Build history of the part. All positions in model axes, mm. A direction names the side the tool comes from. Coordinates: 2 decimals unless noted, no trailing zeros. Loops run counter-clockwise (first coordinate to the right, second up) from the corner with the lowest first, then second, coordinate; pieces in that order, holes last.
Item 1: Cut at D-D (x = 8). List the corners of the cut face in (y, z).
Item 2: Flat gauge pins, fed straight in: pin 1 (1.8 mm diameter, centred on x = 5, z = 10.5, fed in from -Y); pin 2 (5 mm diameter, centred on x = -10.5, y = -11.5, fed in from +Z); pin 3 (8 mm diameter, centred on y = -18.5, z = 16.5, fed in from +X); pin 4 (5.5 mm diameter, centred on x = -4, z = 17, fed in from -Y). Where does each tip first touch, or does it go through?
Item 3: Mould opens along Z. For faces 1 (the face through (-21.53, -2.22, 21.5)), 2 (the face through (-22.5, -10, 14)), 3 (the face through (-4.8, -11.3, 12)), 4 (the face through (-9, -3, 17)) say: released by +Z, released by -Z, zero draft, split by the parting line, or undercut.
Item 4: Drill centre lines: line 1 along Z through (x, y) = (-11, -12); line 2 along Z through (x, y) = (13.5, -1.5); line 3 along Z through (x, y) = (-18.5, -3.25). Where is each one in solid material? Low to high.
Item 5: 3-axis set-ups, long thin cutter, end or side, ignore diameter. For faces 5 (the face through (-14.04, -2.26, 19.67)), 6 (the face through (-12, -3, 24.164)), 7 (the face through (4.31, -14.62, 9.55)), 8 (the face through (-14, -11, 15.164)), 9 (the face through (0, -3, 19)): which of +Z, -Z, +X, -X, +Y, -Y reach the whole face in a straight line?
Item 6: Cut at C-C (z = 16.75). List the corners of the cut face in (x, y), and give its area (3 significant figures).
Item 7: Cut at B-B (y = -14.5). List the corners of the cut face in (x, z).
Item 8: Cut at A-A (x = -16). List the corners of the cut face in (y, z), and give its area (3 significant figures).
from build123d import *

# Parameters (mm, degrees)
F1_DEPTH  = 6
F2_DEPTH  = 23
F3_DEPTH  = 6
F4_R      = 5
F5_W      = 0.81186831
F5_H      = 2
F6_REACH  = 31.1431356237
F8_DEPTH  = 2
F10_DEPTH = 2
F11_R     = 5


with BuildPart() as f1:
    # F0 (on Front) → F1 (new body)
    with BuildSketch(Plane.XZ):
        with BuildLine():
            ThreePointArc((0, 22.7640915698), (-0.4760169509, 23.6848881741), (-1.3951592846, 24.1640915698))
            Line((-1.3951592846, 24.1640915698), (-22.5, 24.1640915698))
            ThreePointArc((-22.5, 24.1640915698), (-21.5061278282, 21.4707603394), (-18.9498743711, 20.1640915698))
            Line((-18.9498743711, 20.1640915698), (-9, 19.1640915698))
            Line((-9, 19.1640915698), (-9, 15.1640915698))
            Line((-9, 15.1640915698), (-6.2313233502, 15.1640915698))
            ThreePointArc((-6.2313233502, 15.1640915698), (-1.9506759829, 13.9418160027), (1.7829414728, 11.5173572715))
            ThreePointArc((1.7829414728, 11.5173572715), (0.6303147693, 13.2130414674), (0, 15.1640915698))
            Line((0, 15.1640915698), (0, 22.7640915698))
        make_face()
    extrude(amount=F1_DEPTH)

    # F0 (on Front) → F2 (join)
    with BuildSketch(Plane.XZ):
        with BuildLine():
            ThreePointArc((2.5376606134, 10.8007404291), (2.1473911285, 11.1454525194), (1.7829414728, 11.5173572715))
            ThreePointArc((1.7829414728, 11.5173572715), (-1.9506759829, 13.9418160027), (-6.2313233502, 15.1640915698))
            Line((-6.2313233502, 15.1640915698), (-9, 15.1640915698))
            Line((-9, 15.1640915698), (-22.5, 15.1640915698))
            Line((-22.5, 15.1640915698), (-22.5, 13.1640915698))
            Line((-22.5, 13.1640915698), (-11, 13.1640915698))
            ThreePointArc((-11, 13.1640915698), (-3.8410894684, 11.591731055), (2, 7.1640915698))
            Line((2, 7.1640915698), (20.2497988939, 7.1640915698))
            Line((20.2497988939, 7.1640915698), (20.2497988939, 9.1640915698))
            Line((20.2497988939, 9.1640915698), (7.4160159886, 9.1640915698))
            ThreePointArc((7.4160159886, 9.1640915698), (7.1261843392, 9.1582804924), (6.8363526899, 9.1640915698))
            Line((6.8363526899, 9.1640915698), (3.930054605, 9.1640915698))
            ThreePointArc((3.930054605, 9.1640915698), (3.2631933631, 10.0073736605), (2.5376606134, 10.8007404291))
        make_face()
    extrude(amount=F2_DEPTH)

    # F0 (on Front) → F3 (join)
    with BuildSketch(Plane.XZ):
        with BuildLine():
            ThreePointArc((6.8363526899, 9.1640915698), (4.5533954509, 9.6314834175), (2.5376606134, 10.8007404291))
            ThreePointArc((2.5376606134, 10.8007404291), (3.2631933631, 10.0073736605), (3.930054605, 9.1640915698))
            Line((3.930054605, 9.1640915698), (6.8363526899, 9.1640915698))
        make_face()
    extrude(amount=F3_DEPTH)

    # F4
    f4_edges = [f1.edges().sort_by_distance(p)[0] for p in [
        (3.930055, -14.5, 9.164092),
    ]]
    fillet(f4_edges, radius=F4_R)

    f6_end = Plane(origin=(-13.9749371855, -3, 19.6640915698), x_dir=(-0.9949874371, 0, 0.1), z_dir=(-0.1, 0, -0.9949874371))
    # F5 (on face) → F6 (cut, up to a plane its end follows)
    with BuildSketch(Plane.XY.offset(24.1640915698)):
        Polygon((-8.5, -6), (-22.5, -4), (-22.5, -6), align=None)
        with Locations((-22.905934155, -5)):
            Rectangle(F5_W, F5_H)
    f6_long = extrude(amount=-F6_REACH, mode=Mode.PRIVATE)
    add(split(f6_long, bisect_by=f6_end, keep=Keep.BOTTOM, mode=Mode.PRIVATE), mode=Mode.SUBTRACT)

    # F7 (on face) → F8 (cut, through all)
    with BuildSketch(Plane.XY.offset(15.1640915698)):
        with BuildLine():
            ThreePointArc((-19.6606274694, -23), (-21.6815784663, -21.9369160005), (-22.5, -19.8051147163))
            Line((-22.5, -19.8051147163), (-22.5, -23))
            Line((-22.5, -23), (-19.6606274694, -23))
        make_face()
    extrude(amount=-F8_DEPTH, mode=Mode.SUBTRACT)

    # F9 (on face) → F10 (cut, through all)
    with BuildSketch(Plane.XY.offset(9.1640915698)):
        with BuildLine():
            ThreePointArc((20.2497988939, -21.1107209325), (19.5387380379, -22.4279634054), (18.1554414653, -23))
            Line((18.1554414653, -23), (20.2497988939, -23))
            Line((20.2497988939, -23), (20.2497988939, -21.1107209325))
        make_face()
    extrude(amount=-F10_DEPTH, mode=Mode.SUBTRACT)

    # F11
    f11_edges = [f1.edges().sort_by_distance(p)[0] for p in [
        (2, -11.5, 7.164092),
    ]]
    fillet(f11_edges, radius=F11_R)


solid = f1.part
Filled sheet:
1. outline: (-23, 7.16) - (0, 7.16) - (0, 9.16) - (-23, 9.16) - close
2. pin 1: passes through
2. pin 2: stops at z = 15.16
2. pin 3: stops at x = 0.55
2. pin 4: stops at y = -23
3. face 1: undercut
3. face 2: zero draft
3. face 3: released by -Z
3. face 4: undercut
4. line 1: z = 13.16 to 15.16
4. line 2: z = 7.16 to 9.16
4. line 3: z = 13.16 to 15.16, 20.12 to 24.16
5. face 5: -X, +Y, -Y
5. face 6: +Z, +X, -X, +Y, -Y
5. face 7: +Z, +X, -Y
5. face 8: -X, -Y
5. face 9: +Z, +X, +Y, -Y
6. outline: (-9, -6) - (0, -6) - (0, 0) - (-9, 0) - close
6. area: 54.0 mm2
7. outline: (-22.5, 13.16) - (-11, 13.16) arc R17.08 cw to (0.71, 8.52) arc R5 ccw to (4.13, 7.16) - (20.25, 7.16) - (20.25, 9.16) - (7.42, 9.16) arc R7.23 cw to (6.84, 9.16) - (6.24, 9.16) arc R5 cw to (2.64, 10.7) arc R15 ccw to (2.54, 10.8) arc R7.23 cw to (1.78, 11.52) arc R15 ccw to (-6.23, 15.16) - (-22.5, 15.16) - close
8. outline: (-23, 13.16) - (0, 13.16) - (0, 15.16) - (-23, 15.16) - close; (-4.93, 19.87) - (0, 19.87) - (0, 24.16) - (-4.93, 24.16) - close
8. area: 67.2 mm2
